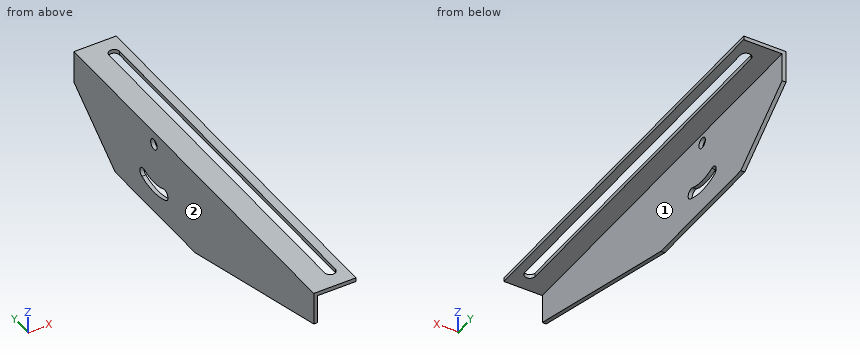
```python
from build123d import *

# Parameters (mm, degrees)
F1_DEPTH = 3
F2_W     = 300
F2_H     = 3
F3_DEPTH = 29
F5_DEPTH = 64.501
F6_R     = 4
F7_DEPTH = 32.001


with BuildPart() as f1:
    # F0 (on Right) → F1 (new body)
    with BuildSketch(Plane.YZ):
        Polygon((150, -25), (150, 0), (-150, 0), (-150, -25), (-1.621217, -64.5), (98.378783, -64.5), align=None)
    extrude(amount=F1_DEPTH)

    # F2 (on face) → F3 (join)
    with BuildSketch(Plane.YZ.offset(3)):
        with Locations((0, -1.5)):
            Rectangle(F2_W, F2_H)
    extrude(amount=F3_DEPTH)

    # F4 (on face) → F5 (cut, through all)
    with BuildSketch(Plane.XY):
        with BuildLine():
            ThreePointArc((17.4, -135), (21.4, -139), (25.4, -135))
            Line((25.4, -135), (25.4, 135))
            ThreePointArc((25.4, 135), (21.4, 139), (17.4, 135))
            Line((17.4, 135), (17.4, -135))
        make_face()
    extrude(amount=-F5_DEPTH, mode=Mode.SUBTRACT)

    # F6 (on face) → F7 (cut, through all)
    with BuildSketch(Plane(origin=(0, 0, 0), x_dir=(0, -1, 0), z_dir=(-1, 0, 0))):
        with Locations((-50, -10)):
            Circle(F6_R)
        with BuildLine():
            ThreePointArc((-61.957143, -38.601167), (-67.190473, -40.748783), (-65.042857, -45.982113))
            ThreePointArc((-65.042857, -45.982113), (-50, -49), (-34.957143, -45.982113))
            ThreePointArc((-34.957143, -45.982113), (-32.809527, -40.748783), (-38.042857, -38.601167))
            ThreePointArc((-38.042857, -38.601167), (-50, -41), (-61.957143, -38.601167))
        make_face()
    extrude(amount=-F7_DEPTH, mode=Mode.SUBTRACT)


solid = f1.part
```
Here's how the part is built. I have some questions about the finished solid (model axes, mm). Face numbers are marked on the shaded views. A direction names the side the tool comes from. Give positions to 0.01 mm unless a question says otherwise; leave off trailing zeros. Order: outer loops, then holes, each group sorted by start corner. A loop starts at its lowest first (then second) coordinate and runs counter-clockwise, first axis right, second up. Notation, with made-up numbers: M 53.25,-3.75 L 75.25,-3.75 A11 ccw 75.25,8.25 Z; hole C 48.25,74.5 d6. An arc over 180 degrees is marked long. Use a Markdown table: item, result. Add a question column.
1. On a 3-axis mill with a long thin cutter (end or side, diameter ignored), from which of +Z, -Z, +X, -X, +Y, -Y can I reach the whole of each face in a straight line? I mean the marked faces 1 and 2. Say none if no direction works.
2. I need wall thicknesses on probe 1 along Z at (x, y) = (1, 50); probe 2 along X at (y, z) = (-1, -21); probe 3 along Z at (x, y) = (25.5, 127). Which ranges of each line are inside material? Lowest first, please. Write a range as from..to.
3. Suppose I cut it at C-C (y = 88.5). List the corners of the cut face in (x, z) for me, and give its area (4 significant figures).
4. Suppose I cut it at B-B (y = 50). List the corners of the cut face in (x, z) for me.
5. Suppose I cut it at D-D (y = -71.5). List the corners of the cut face in (x, z) for me.
6. For pin 1 Ø1 at (y, z) = (31, -44) entering from +X; pin 2 Ø6 at (x, y) = (25.5, 38.5) entering from -Z, each with a flat end and sliding along its axis, tell me the tip position at first contact or that it passes through.
7. Suppose I cut it at A-A (z = -10). List the corners of the cut face in (x, y) for me.
Results list:
| question | item | result |
|---|---|---|
| 1 | face 1 | -Z, +X, +Y, -Y |
| 1 | face 2 | +Z, -Z, -X, +Y, -Y |
| 2 | probe 1 | z = -64.5..-49, -41..-14, -6..0 |
| 2 | probe 2 | x = 0..3 |
| 2 | probe 3 | z = -3..0 |
| 3 | outline | M 0,-64.5 L 3,-64.5 L 3,-3 L 17.4,-3 L 17.4,0 L 0,0 Z; M 25.4,-3 L 32,-3 L 32,0 L 25.4,0 Z |
| 3 | area | 256.5 mm² |
| 4 | outline | M 0,-64.5 L 3,-64.5 L 3,-49 L 0,-49 Z; M 0,-41 L 3,-41 L 3,-14 L 0,-14 Z; M 0,-6 L 3,-6 L 3,-3 L 17.4,-3 L 17.4,0 L 0,0 Z; M 25.4,-3 L 32,-3 L 32,0 L 25.4,0 Z |
| 5 | outline | M 0,-45.9 L 3,-45.9 L 3,-3 L 17.4,-3 L 17.4,0 L 0,0 Z; M 25.4,-3 L 32,-3 L 32,0 L 25.4,0 Z |
| 6 | pin 1 | stops at x = 3 |
| 6 | pin 2 | stops at z = -3 |
| 7 | outline | M 0,-150 L 3,-150 L 3,46 L 0,46 Z; M 0,54 L 3,54 L 3,150 L 0,150 Z |
